Model file for the job. Use its own axes, mm. A direction names the side the tool comes from. Coordinates: 2 decimals unless noted, no trailing zeros. Write each loop counter-clockwise with the first axis right and the second up, starting at its lowest first coordinate (ties: lowest second). Pieces come first, ordered by that corner, then holes. Notation, with made-up numbers: (72, 57.5) -> (83, 57.5) arc R9 ccw to (83, 70.5) -> close; hole circle Ø1 at (-27.5, -1.5). An arc over 180 degrees is marked (long way). Answer as a JSON object with one key per item and string values. Group by question number.
from build123d import *

# Parameters (mm, degrees)
F0_R          = 22
F1_DEPTH      = 32
F2_W          = 14.3667660505
F2_H          = 12.7565913796
F2_W_2        = 13.8227823973
F2_H_2        = 11.8480638564
F3_DEPTH      = 22.001
F3_DEPTH_BACK = 25
F4_W          = 16.210654363
F4_H          = 15.0942654014
F4_W_2        = 16.4447609186
F4_H_2        = 12.1968873441
F5_DEPTH      = 22.001
F5_DEPTH_BACK = 25
F6_SIZE       = 1


with BuildPart() as f1:
    # F0 (on Top) → F1 (new body)
    with BuildSketch(Plane.XY):
        Circle(F0_R)
    extrude(amount=F1_DEPTH)

    # F2 (on Front) → F3 (cut, two sides)
    with BuildSketch(Plane.XZ) as f3_sk:
        with Locations((-16.1833830252, 27.3782956898)):
            Rectangle(F2_W, F2_H)
        with Locations((15.9113911986, 26.9240319282)):
            Rectangle(F2_W_2, F2_H_2)
    extrude(amount=F3_DEPTH, mode=Mode.SUBTRACT)
    extrude(f3_sk.sketch, amount=-F3_DEPTH_BACK, mode=Mode.SUBTRACT)

    # F4 (on Right) → F5 (cut, two sides)
    with BuildSketch(Plane.YZ) as f5_sk:
        with Locations((-17.1053271815, 3.4528672993)):
            Rectangle(F4_W, F4_H)
        with Locations((17.2223804593, 4.9015563279)):
            Rectangle(F4_W_2, F4_H_2)
    extrude(amount=-F5_DEPTH, mode=Mode.SUBTRACT)
    extrude(f5_sk.sketch, amount=F5_DEPTH_BACK, mode=Mode.SUBTRACT)

    # F6
    f6_edges = [f1.edges().sort_by_distance(p)[0] for p in [
        (9, 0, 32),
        (0, -22, 32),
        (-9, 0, 32),
        (0, 22, 32),
        (21.513332, -4.601798, 0),
        (0, -9, 0),
        (-22, 0, 0),
        (0, 9, 0),
        (21.513332, 4.601798, 0),
    ]]
    chamfer(f6_edges, length=F6_SIZE)


solid = f1.part
(1) Cut at B-B on y = 0. List the corners of the cut face in (x, z), plus the area to 3 significant figures.
(2) Cut at A-A on x = 0. List the corners of the cut face in (y, z).
(3) Cut at C-C on z = 8. List the corners of the cut face in (x, y), plus the area to 3 significant figures.
(4) Cut at D-D on y = 15. List the corners of the cut face in (x, z).
(5) 3-axis set-ups, long thin cutter, end or side, ignore diameter. For faces 1 (the face through (0, 14, 11)), 2 (the face through (21.2, -0.1, 0.2)), 3 (the face through (14, 0, 21)), 4 (the face through (-9, 0, 26)), 5 (the face through (0, -9, 6)): which of +Z, -Z, +X, -X, +Y, -Y reach the whole face in a straight line?
(6) Wall check: probe 1 along X at (y, z) = (-15.5, 22); probe 2 along Z at (x, y) = (15, -14). Give the ranges that are in metal, low to high.
(7) Pin check, flat tips, straight feed: pin 1 (3 mm diameter, centred on x = 4, z = 25, fed in from -Y); pin 2 (3 mm diameter, centred on x = -11, y = -9.5, fed in from +Z); pin 3 (11 mm diameter, centred on x = -7.5, z = 8, fed in from +Y). Stop position of each tip, or through.
Results found:
{
 "1": {"outline": "(-22, 1) -> (-21, 0) -> (21, 0) -> (22, 1) -> (22, 21) -> (9, 21) -> (9, 31) -> (8, 32) -> (-8, 32) -> (-9, 31) -> (-9, 21) -> (-22, 21) -> close", "area": "1,120 mm²"},
 "2": {"outline": "(-22, 11) -> (-9, 11) -> (-9, 1) -> (-8, 0) -> (8, 0) -> (9, 1) -> (9, 11) -> (22, 11) -> (22, 31) -> (21, 32) -> (-21, 32) -> (-22, 31) -> close"},
 "3": {"outline": "(-20.07, -9) -> (20.07, -9) arc R22 ccw to (20.07, 9) -> (-20.07, 9) arc R22 ccw to start", "area": "769 mm²"},
 "4": {"outline": "(-16.09, 11) -> (16.09, 11) -> (16.09, 21) -> (9, 21) -> (9, 31) -> (8, 32) -> (-8, 32) -> (-9, 31) -> (-9, 21) -> (-16.09, 21) -> close"},
 "5": {"face 1": "-Z, +X, -X, +Y", "face 2": "-Z, +X", "face 3": "+Z, +X, +Y, -Y", "face 4": "+Z, -X, +Y, -Y", "face 5": "-Z, +X, -X, -Y"},
 "6": {"probe 1": "x = -9 to 9", "probe 2": "z = 11 to 21"},
 "7": {"pin 1": "stops at y = -21.86", "pin 2": "stops at z = 21", "pin 3": "stops at y = 21.81"}
}
